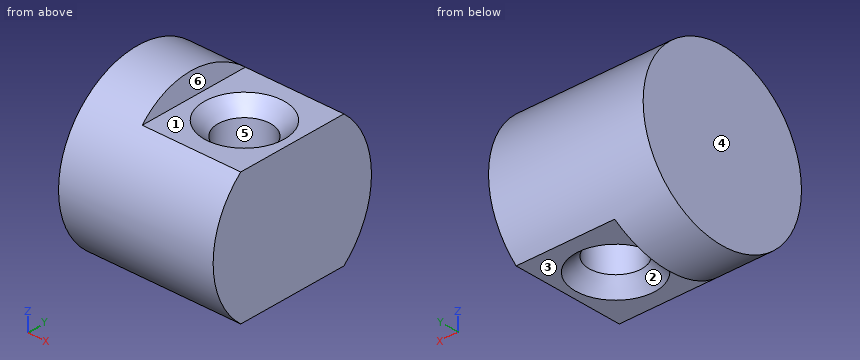
```python
from build123d import *

# Parameters (mm, degrees)
F0_R          = 8.001
F1_DEPTH      = 14.351
F3_DEPTH      = 25.4
F3_DEPTH_BACK = 25.4
F4_R          = 2.4384
F5_DEPTH      = 25.4
F5_DEPTH_BACK = 25.4
F6_SIZE       = 1.27


with BuildPart() as f1:
    # F0 (on Right) → F1 (new body)
    with BuildSketch(Plane.YZ):
        Circle(F0_R)
    extrude(amount=F1_DEPTH)

    # F2 (on Front) → F3 (cut, two sides)
    with BuildSketch(Plane.XZ) as f3_sk:
        Polygon((14.351, 8.001), (4.953, 8.001), (5.207, 6.0706), (14.351, 6.0706), align=None)
        Polygon((4.953, -8.001), (14.351, -8.001), (14.351, -6.0706), (5.207, -6.0706), align=None)
    extrude(amount=-F3_DEPTH, mode=Mode.SUBTRACT)
    extrude(f3_sk.sketch, amount=F3_DEPTH_BACK, mode=Mode.SUBTRACT)

    # F4 (on Top) → F5 (cut, two sides)
    with BuildSketch(Plane.XY) as f5_sk:
        with Locations((9.906, 0)):
            Circle(F4_R)
    extrude(amount=-F5_DEPTH, mode=Mode.SUBTRACT)
    extrude(f5_sk.sketch, amount=F5_DEPTH_BACK, mode=Mode.SUBTRACT)

    # F6
    f6_edges = [f1.edges().sort_by_distance(p)[0] for p in [
        (7.4676, 0, 6.0706),
        (7.4676, 0, -6.0706),
    ]]
    chamfer(f6_edges, length=F6_SIZE)


solid = f1.part
```
CAD build for the part. Positions are in the model's coordinates, mm. Face numbers are marked on the shaded views. A direction names the side the tool comes from. Round coordinates to 2 decimals unless told otherwise and drop trailing zeros. Write each loop counter-clockwise with the first axis right and the second up, starting at its lowest first coordinate (ties: lowest second). Pieces come first, ordered by that corner, then holes. Notation, with made-up numbers: (-21.5, 77) - (4.5, 77) arc R28 ccw to (4.5, 99) - close; hole circle Ø8 at (35, -32.5). An arc over 180 degrees is marked (long way). Return JSON: item names as keys, results as strings. Group by question number.
Item 1: Band-saw the part on C-C on x = 3.5. List the corners of the cut face in (y, z).
Item 2: Probe probe 1 along X at (y, z) = (0, -2); probe 2 along Z at (x, y) = (12.5, 4.75); probe 3 along Y at (x, z) = (9.25, -2.25). List the from-to ranges inside material, lowest first.
Item 3: Band-saw the part on B-B on z = 0. List the corners of the cut face in (x, y), plus the area to 3 significant figures.
Item 4: Flat gauge pins, fed straight in: pin 1 Ø1 at (x, z) = (9, -1.5) entering from -Y; pin 2 Ø4 at (x, z) = (11, -3.5) entering from +Y; pin 3 Ø4 at (x, y) = (9.906, 0) entering from -Z; pin 4 Ø8 at (x, y) = (9.5, -1.5) entering from +Z. Where does each tip first touch, or does it go through?
Item 5: Band-saw the part on D-D on y = -4. List the corners of the cut face in (x, z).
Item 6: Mould opens along X. For the marked faces 3, 4, 5 and 6 say: +X half, -X half, draft (parallel to the pull), parting line (faces both ways), or undercut.
Item 7: 3-axis set-ups, long thin cutter, end or side, ignore diameter. For the marked faces 1 and 2: which of +Z, -Z, +X, -X, +Y, -Y reach the whole face in a straight line?
Item 8: Band-saw the part on A-A on y = 0. List the corners of the cut face in (x, z), plus the area to 3 significant figures.
Resolved:
{
 "1": {"outline": "circle Ø16 at (0, 0)"},
 "2": {"probe 1": "x = 0 to 7.47, 12.34 to 14.35", "probe 2": "z = -6.07 to 6.07", "probe 3": "y = -7.68 to -2.35, 2.35 to 7.68"},
 "3": {"outline": "(0, -8) - (14.35, -8) - (14.35, 8) - (0, 8) - close; hole circle Ø4.88 at (9.91, 0)", "area": "211 mm²"},
 "4": {"pin 1": "stops at y = -7.94", "pin 2": "stops at y = 7.86", "pin 3": "passes through", "pin 4": "stops at z = 6.07"},
 "5": {"outline": "(0, -6.93) - (5.09, -6.93) - (5.21, -6.07) - (14.35, -6.07) - (14.35, 6.07) - (5.21, 6.07) - (5.09, 6.93) - (0, 6.93) - close"},
 "6": {"face 3": "draft", "face 4": "-X half", "face 5": "undercut", "face 6": "+X half"},
 "7": {"face 1": "+Z, +X, +Y, -Y", "face 2": "-Z"},
 "8": {"outline": "(0, -8) - (4.95, -8) - (5.21, -6.07) - (6.2, -6.07) - (7.47, -4.8) - (7.47, 4.8) - (6.2, 6.07) - (5.21, 6.07) - (4.95, 8) - (0, 8) - close; (12.34, -4.8) - (13.61, -6.07) - (14.35, -6.07) - (14.35, 6.07) - (13.61, 6.07) - (12.34, 4.8) - close", "area": "131 mm²"}
}
